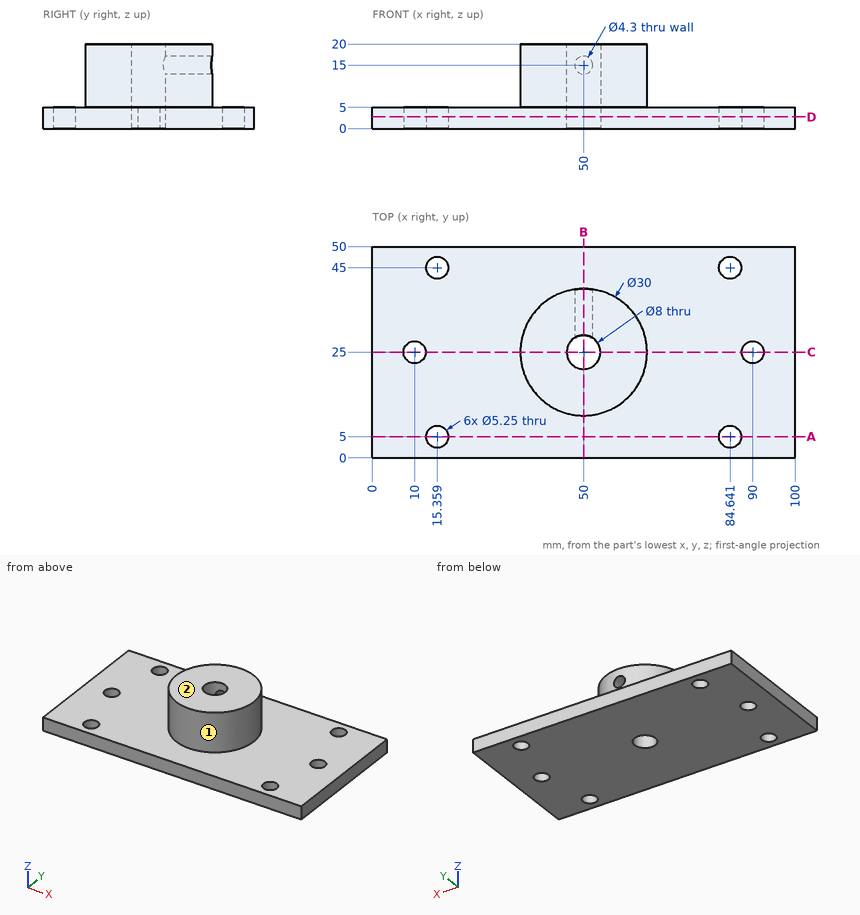
Print and shaded views of the part. All mm, measured from the part's lowest x, y and z. A direction names the side the tool comes from. Give positions to 0.01 mm unless a question says otherwise; leave off trailing zeros. Loops run counter-clockwise (first coordinate to the right, second up) from the corner with the lowest first, then second, coordinate; pieces in that order, holes last.
1) Saw through at C-C (y = 25). Write the cut outline in (x, z) (3 decimals).
2) Wall check: line 1 (Y direction, x = 90, z = 2.7) (3 decimals); line 2 (Z direction, x = 81, y = 44); line 3 (X direction, y = 24.5, z = 18.25). Give the ranges that are in metal, low to high.
3) Tool access for the marked faces 1 and 2: list every direction of +Z, -Z, +X, -X, +Y, -Y with a clear straight run to the whole face (end or side of a thin tool).
4) Saw through at A-A (y = 5). Write the cut outline in (x, z).
5) Saw through at D-D (z = 2.75). Write the cut outline in (x, y) (3 decimals).
6) Saw through at B-B (x = 50). Write the cut outline in (y, z).
7) Flat gauge pins, fed straight in: pin 1 Ø7 at (x, z) = (50, 15) entering from -Y; pin 2 Ø4.5 at (x, y) = (84.64, 45) entering from +Z; pin 3 Ø4 at (y, z) = (40.5, 10) entering from -X; pin 4 Ø7 at (x, y) = (15.36, 5) entering from +Z. Where does each tip first touch, or does it go through?
Answer block:
1. outline: (0, 0) - (7.375, 0) - (7.375, 5) - (0, 5) - close; (12.625, 0) - (46, 0) - (46, 20) - (35, 20) - (35, 5) - (12.625, 5) - close; (54, 0) - (87.375, 0) - (87.375, 5) - (65, 5) - (65, 20) - (54, 20) - close; (92.625, 0) - (100, 0) - (100, 5) - (92.625, 5) - close
2. line 1: y = 0 to 22.375, 27.625 to 50
2. line 2: z = 0 to 5
2. line 3: x = 35.01 to 46.03, 53.97 to 64.99
3. face 1: +Z
3. face 2: +Z, +X, -X, +Y, -Y
4. outline: (0, 0) - (12.73, 0) - (12.73, 5) - (0, 5) - close; (17.98, 0) - (82.02, 0) - (82.02, 5) - (17.98, 5) - close; (87.27, 0) - (100, 0) - (100, 5) - (87.27, 5) - close
5. outline: (0, 0) - (100, 0) - (100, 50) - (0, 50) - close; hole circle Ø5.25 at (10, 25); hole circle Ø5.25 at (15.359, 5); hole circle Ø5.25 at (15.359, 45); hole circle Ø8 at (50, 25); hole circle Ø5.25 at (84.641, 5); hole circle Ø5.25 at (84.641, 45); hole circle Ø5.25 at (90, 25)
6. outline: (0, 0) - (21, 0) - (21, 20) - (10, 20) - (10, 5) - (0, 5) - close; (29, 0) - (50, 0) - (50, 5) - (40, 5) - (40, 12.85) - (29, 12.85) - close; (29, 17.15) - (40, 17.15) - (40, 20) - (29, 20) - close
7. pin 1: stops at y = 10
7. pin 2: passes through
7. pin 3: stops at x = 43.46
7. pin 4: stops at z = 5
